The model under review builds one solid part; all positions refer to its coordinate system, in mm. A direction names the side the tool comes from. Give positions to 0.01 mm unless a question says otherwise; leave off trailing zeros. Loops run counter-clockwise (first coordinate to the right, second up) from the corner with the lowest first, then second, coordinate; pieces in that order, holes last. Notation, with made-up numbers: M -23.75,-10.5 L 33.25,-10.5 A19 cw 33.25,6.5 Z; hole C 53.25,7 d4. An arc over 180 degrees is marked long. Return JSON: item names as keys, results as strings. Group by question number.
```python
from build123d import *

# Parameters (mm, degrees)
SKETCH1_R                = 20
SKETCH1_R_2              = 16
BOSS_EXTRUDE1_DEPTH      = 430
BOSS_EXTRUDE2_REACH      = 438.119
BOSS_EXTRUDE2_END_RADIUS = 20
SKETCH2_W                = 25
SKETCH2_H                = 5
FILLET1_R                = 10
SKETCH3_R                = 6.5
CUT_EXTRUDE1_DEPTH       = 10


with BuildPart() as part:
    # Sketch1 → Boss-Extrude1 (new body)
    with BuildSketch(Plane(origin=(0, 0, 0), x_dir=(0, 0, -1), z_dir=(1, 0, 0))):
        Circle(SKETCH1_R)
        Circle(SKETCH1_R_2, mode=Mode.SUBTRACT)
    extrude(amount=-BOSS_EXTRUDE1_DEPTH)

    # Boss-Extrude2: up to this cylinder (the profile starts outside it)
    boss_extrude2_end = Plane(origin=(-42.5, 0, 0), z_dir=(1, 0, 0)) * Cylinder(BOSS_EXTRUDE2_END_RADIUS, 917.238, mode=Mode.PRIVATE)
    # Sketch2 → Boss-Extrude2 (add, up to the surface)
    with BuildSketch(Plane(origin=(0, 50, 0), x_dir=(1, 0, 0), z_dir=(0, 1, 0)), mode=Mode.PRIVATE) as boss_extrude2_sk1:
        with Locations((-42.5, 0)):
            Rectangle(SKETCH2_W, SKETCH2_H)
    boss_extrude2_tool1 = extrude(boss_extrude2_sk1.sketch, amount=-BOSS_EXTRUDE2_REACH, mode=Mode.PRIVATE) - boss_extrude2_end
    add(boss_extrude2_tool1.solids().sort_by_distance((-42.5, 50, 0))[0])

    # Fillet1
    fillet1_edges = [part.edges().sort_by_distance(p)[0] for p in [
        (-30, 50, 0),
        (-55, 50, 0),
    ]]
    fillet(fillet1_edges, radius=FILLET1_R)

    # Sketch3 → Cut-Extrude1 (cut)
    with BuildSketch(Plane.XY.offset(2.5)):
        with Locations((-42.5, 37)):
            Circle(SKETCH3_R)
    extrude(amount=-CUT_EXTRUDE1_DEPTH, mode=Mode.SUBTRACT)


solid = part.part
```
(1) Add section C-C (x = -280.5). Write out the cut boundary in (y, z).
(2) Mouldability with a two-part tool opening along X and no side actions: class faces 1 (the cylindrical face through (-52.15, 46.99, -0.04)), 2 (the cylindrical face through (-49, 37, 0)), 3 (the flat face through (-43, 28, -2.5)) as released by +X, released by -X, zero draft, split by the parting line, or undercut.
(3) For faces 4 (the flat face through (-430, 13.43, 8.98)), 5 (the flat face through (-43, 28, 2.5)), list the 3-axis set-ups (+Z, -Z, +X, -X, +Y, -Y) from which the entire face can be reached by the end or side of a thin tool; tool diameter is ignored.
(4) For probe 1 along Y at (x, z) = (-191.5, 0); probe 2 along Z at (x, y) = (-244.5, -2.5); probe 3 along Y at (x, z) = (-146.5, 13.5), list the stretches that pass through material, from the lowest coordinate up.
(5) For pin 1 (1 mm diameter, centred on x = -218, y = -9.5, fed in from -Z); pin 2 (4 mm diameter, centred on x = -247.5, z = 9.5, fed in from +Y); pin 3 (15 mm diameter, centred on x = -42.5, y = 37, fed in from -Z), all flat-tipped, find the tip position at first contact; note any pin that passes through.
(6) Add section A-A (y = 0). Write out the cut boundary in (x, z), and give its area (3 significant figures).
(7) Add section B-B (z = -6). Write out the cut boundary in (x, y), and give its area (3 significant figures).
Verdict:
{
 "1": {"outline": "C 0,0 d40; hole C 0,0 d32"},
 "2": {"face 1": "released by -X", "face 2": "undercut", "face 3": "zero draft"},
 "3": {"face 4": "+Z, -Z, -X, +Y, -Y", "face 5": "+Z, +X, -X, +Y"},
 "4": {"probe 1": "y = -20 to -16, 16 to 20", "probe 2": "z = -19.84 to -15.8, 15.8 to 19.84", "probe 3": "y = -14.76 to -8.59, 8.59 to 14.76"},
 "5": {"pin 1": "stops at z = -17.86", "pin 2": "stops at y = 18.54", "pin 3": "stops at z = -2.5"},
 "6": {"outline": "M -430,-20 L 0,-20 L 0,-16 L -430,-16 Z; M -430,16 L 0,16 L 0,20 L -430,20 Z", "area": "3,440 mm²"},
 "7": {"outline": "M -430,-19.08 L 0,-19.08 L 0,-14.83 L -430,-14.83 Z; M -430,14.83 L 0,14.83 L 0,19.08 L -430,19.08 Z", "area": "3,650 mm²"}
}
